Autodesk Inventor part; units mm, degrees
ref_plane "YZ Plane" through (0, 0, 0) normal (1, 0, 0) x (0, 1, 0)
ref_plane "XZ Plane" through (0, 0, 0) normal (0, 1, 0) x (-1, 0, 0)
ref_plane "XY Plane" through (0, 0, 0) normal (0, 0, 1) x (1, 0, 0)
sketch "Sketch1" plane through (0, 0, 0) normal (0, 1, 0) x (-1, 0, 0)
  line L0 (10, 10) -> (-10, 10)
  line L1 (-10, 10) -> (-10, -10)
  line L2 (-10, -10) -> (10, -10)
  line L3 (10, -10) -> (10, 10)
  line L4 (10, 10) -> (-10, -10) construction
  line L5 (-10, 10) -> (10, -10) construction
  point P0 (0, 0)
  dimension "d0" = 20
  dimension "d1" = 20
extrude "Extrusion1" add sketch "Sketch1" along normal blind 75
sketch "Sketch2" plane through (0, 75, 0) normal (0, 1, 0) x (1, 0, 0)
  circle A0 centre (-1.5, 0) radius 4.6
  line L0 (-10, -10) -> (10, -10)
  line L1 (-10, 10) -> (-10, -10)
  dimension "d4" = 9.2
  dimension "d25" = 10
  dimension "d26" = 8.5
extrude "Extrusion2" cut sketch "Sketch2" against normal blind 10
sketch "Sketch3" plane through (0, 0, 0) normal (0, -1, 0) x (1, 0, 0)
  circle A0 centre (-1.5, 0) radius 7.5
  line L0 (10, -10) -> (-10, -10)
  line L1 (-10, -10) -> (-10, 10)
  dimension "d7" = 15
  dimension "d27" = 10
  dimension "d28" = 8.5
extrude "Extrusion3" cut sketch "Sketch3" against normal blind 65
sketch "Sketch5" plane through (10, 0, 10) normal (1, 0, 0) x (0, 0, -1)
  line L0 (20, 75) -> (0, 75)
  line L1 (0, 75) -> (0, 0)
  line L2 (0, 0) -> (20, 0)
  line L3 (20, 0) -> (20, 75)
  line L4 (20, 0) -> (20, 75)
  line L5 (0, 0) -> (20, 0)
  line L6 (0, 75) -> (20, 75)
  line L7 (0, 0) -> (0, 75)
  point P0 (10, 0)
extrude "Extrusion5" add sketch "Sketch5" along normal blind 5
sketch "Sketch7" plane through (-10, 0, -10) normal (0, 0, -1) x (-1, 0, 0)
  circle A0 centre (-21, 55) radius 1.55
  circle A1 centre (-21, 40) radius 1.55
  circle A2 centre (-21, 25) radius 1.55
  line L0 (0, 75) -> (-25, 75)
  line L1 (-25, 0) -> (-25, 75)
  point P0 (-10, 0)
  dimension "d16" = 3.1
  dimension "d17" = 3.1
  dimension "d18" = 3.1
  dimension "d19" = 20
  dimension "d20" = 15
  dimension "d21" = 15
  dimension "d22" = 4
extrude "Extrusion6" cut sketch "Sketch7" against normal blind 20
sketch "Sketch8" plane through (-10, 0, -10) normal (0, 0, -1) x (-1, 0, 0)
  line L0 (-17, 75) -> (-25, 75)
  line L1 (-25, 75) -> (-25, 15)
  line L2 (-25, 15) -> (-17, 15)
  line L3 (-17, 15) -> (-17, 75)
  line L4 (0, 0) -> (-25, 0)
  line L5 (0, 75) -> (-25, 75)
  line L6 (-25, 0) -> (-25, 75)
  point P0 (-10, 0)
  dimension "d29" = 8
  dimension "d32" = 15
extrude "Extrusion7" cut sketch "Sketch8" against normal blind 8
sketch "Sketch9" plane through (-10, 0, -10) normal (0, 0, -1) x (-1, 0, 0)
  circle A0 centre (-8.1, 5) radius 1.55
  line L0 (0, 0) -> (0, 75)
  line L1 (0, 0) -> (-25, 0)
  point P0 (-10, 0)
  dimension "d33" = 3.1
  dimension "d34" = 8.1
  dimension "d35" = 5
extrude "Extrusion8" cut sketch "Sketch9" against normal through all
sketch "Sketch10" plane through (0, 0, 0) normal (0, -1, 0) x (1, 0, 0)
  line L0 (15, -10) -> (10, -10)
  line L1 (10, -10) -> (10, 10)
  line L2 (10, 10) -> (15, 10)
  line L3 (15, 10) -> (15, -10)
  line L4 (-10, -10) -> (15, -10)
  line L5 (-10, 10) -> (15, 10)
  line L6 (15, 10) -> (15, -10)
  point P0 (0, 0)
  dimension "d38" = 5
extrude "Extrusion9" add sketch "Sketch10" along normal blind 5
fillet "Fillet1" radius 2 17 edges at (15, 35, 10) (-10, 37.5, 10) (15, 45, -2) (7, 45, -10) (-10, 37.5, -10) (-1.5, 75, -10) (7, 75, -6) (11, 75, -2) (15, 75, 4) (2.5, 75, 10) (-10, 75, 0) (11, 15, -10) (15, 15, -6) (15, 5, -10) (15, -5, 0) (12.5, -5, -10) (12.5, -5, 10)
properties part number "finger2" material "ABS Plastic"
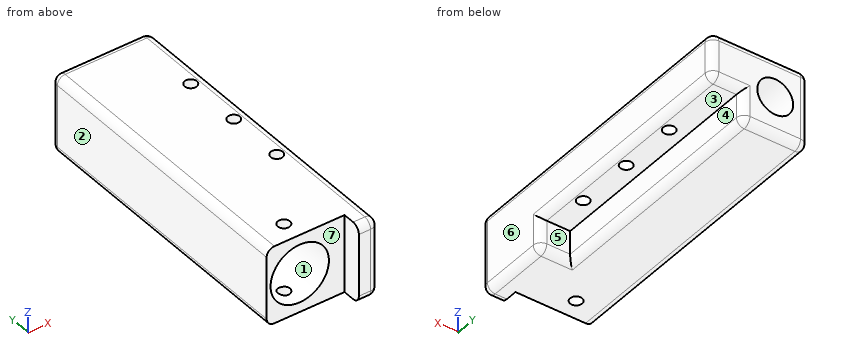
The listing builds one solid part. Answer for the finished solid, in the listing's coordinates (mm). Face numbers are marked on the shaded views. A direction names the side the tool comes from. Give positions to 0.01 mm unless a question says otherwise; leave off trailing zeros. Write each loop counter-clockwise with the first axis right and the second up, starting at its lowest first coordinate (ties: lowest second). Pieces come first, ordered by that corner, then holes. Notation, with made-up numbers: (51.25, 0.5) -> (107.25, 0.5) arc R30 ccw to (107.25, 34.5) -> close; hole circle Ø6 at (23, -34). An arc over 180 degrees is marked (long way). Write item = value, one per line. Start each with the question number.
1) The part is cut by section C-C, the plane y = 60. Determine the outline of the cut face in (x, z).
2) Which of the six approach directions +Z, -Z, +X, -X, +Y, -Y give full straight-line access (tool end or side, diameter ignored) to the marked faces 5, 6 and 7?
3) The part is cut by section B-B, the plane x = -1.5. Determine the outline of the cut face in (y, z).
4) The part is cut by section A-A, the plane y = 25. Determine the outline of the cut face in (x, z), and give its area (3 significant figures).
5) Each of these flat-tipped pins is pushed along its axis until it touches: pin 1 (12 mm diameter, centred on x = -2.5, z = 1, fed in from -Y); pin 2 (5.5 mm diameter, centred on y = -3, z = -5, fed in from -X); pin 3 (6.5 mm diameter, centred on x = 11, z = -4.5, fed in from +Y). Where does it stop, or does it pass through?
6) The part is cut by section D-D, the plane z = -5.5. Determine the outline of the cut face in (x, y), and give its area (3 significant figures).
7) Determine the mould class of the marked faces 1, 2, 3 and 4 for opening direction X: +X half, -X half, draft (parallel to the pull), parting line (faces both ways), or undercut.
8) Straight lines are drawn through the part: line 1 along Y through (x, z) = (11, 6.75); line 2 along X through (y, z) = (72, 0); line 3 along Z through (x, y) = (-2, 42.5). For each, find the intervals that lie inside material, in ascending order.
Solutions:
q1.outline = (-10, -8) arc R2 ccw to (-8, -10) -> (5, -10) arc R2 ccw to (7, -8) -> (7, -2) -> (13, -2) arc R2 ccw to (15, 0) -> (15, 8) arc R2 ccw to (13, 10) -> (-8, 10) arc R2 ccw to (-10, 8) -> close; hole circle Ø15 at (-1.5, 0)
q2.face_5 = -Z, +X, +Y
q2.face_6 = +Z, -Z, +X, +Y, -Y
q2.face_7 = +Z, -Z, -X, -Y
q3.outline = (0, -10) -> (3.5, -10) -> (3.5, -7.5) -> (0, -7.5) -> close; (0, 7.5) -> (3.5, 7.5) -> (3.5, 10) -> (0, 10) -> close; (6.5, -10) -> (73, -10) arc R2 ccw to (75, -8) -> (75, -4.6) -> (65, -4.6) -> (65, -7.5) -> (6.5, -7.5) -> close; (6.5, 7.5) -> (65, 7.5) -> (65, 4.6) -> (75, 4.6) -> (75, 8) arc R2 ccw to (73, 10) -> (6.5, 10) -> close
q4.outline = (-10, -8) arc R2 ccw to (-8, -10) -> (5, -10) arc R2 ccw to (7, -8) -> (7, -2) -> (9.45, -2) -> (9.45, 10) -> (-8, 10) arc R2 ccw to (-10, 8) -> close; (12.55, -2) -> (13, -2) arc R2 ccw to (15, 0) -> (15, 8) arc R2 ccw to (13, 10) -> (12.55, 10) -> close; hole circle Ø15 at (-1.5, 0)
q4.area = 218 mm²
q5.pin_1 = 65
q5.pin_2 = 10
q5.pin_3 = 74.56
q6.outline = (-10, 0) -> (-6.6, 0) -> (-6.6, 65) -> (3.6, 65) -> (3.6, 0) -> (10, 0) -> (10, -5) -> (13, -5) arc R2 ccw to (15, -3) -> (15, 13) arc R2 ccw to (13, 15) -> (7, 15) -> (7, 73) arc R2 ccw to (5, 75) -> (-8, 75) arc R2 ccw to (-10, 73) -> close
q6.area = 754 mm²
q7.face_1 = undercut
q7.face_2 = -X half
q7.face_3 = draft
q7.face_4 = +X half
q8.line_1 = -5 to 23.45, 26.55 to 38.45, 41.55 to 53.45, 56.55 to 75
q8.line_2 = -10 to -6.1, 3.1 to 15
q8.line_3 = -10 to -7.48, 7.48 to 10
